```python
from build123d import *

# Parameters (mm, degrees)
BOSS_EXTRUDE1_DEPTH = 50
SKETCH2_W           = 20
SKETCH2_H           = 40
CUT_EXTRUDE1_DEPTH  = 50


with BuildPart() as part:
    # Sketch1 → Boss-Extrude1 (new body)
    with BuildSketch(Plane(origin=(0, 0, 0), x_dir=(1, 0, 0), z_dir=(0, 1, 0))):
        Polygon((40, -2.5), (40, 0), (40, 2.5), (-40, 2.5), (-40, -2.5), align=None)
    extrude(amount=BOSS_EXTRUDE1_DEPTH)

    # Sketch2 → Cut-Extrude1 (cut)
    with BuildSketch(Plane.XY.offset(2.5)):
        with Locations((10, 30)):
            Rectangle(SKETCH2_W, SKETCH2_H)
        with Locations((-10, 30)):
            Rectangle(SKETCH2_W, SKETCH2_H)
    extrude(amount=-CUT_EXTRUDE1_DEPTH, mode=Mode.SUBTRACT)


solid = part.part
```
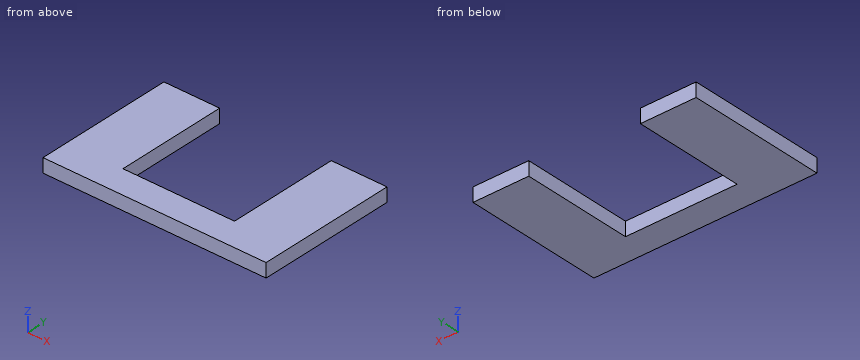
Design review of the part built by this model. Coordinates are the model's own, in mm. Round coordinates to 2 decimals unless told otherwise and drop trailing zeros. Write each loop counter-clockwise with the first axis right and the second up, starting at its lowest first coordinate (ties: lowest second). Pieces come first, ordered by that corner, then holes. Notation, with made-up numbers: (-25.5, -6.75) -> (20.5, -6.75) arc R17 cw to (20.5, -0.75) -> close; hole circle Ø1 at (84.25, 29). An arc over 180 degrees is marked (long way). Answer in a Markdown table with one row per item.
Q1. Take a section at C-C, the plane x = 3. State the section outline as (y, z) points, then the cut area to 3 significant figures.
The answers:
| item | result |
|---|---|
| outline | (0, -2.5) -> (10, -2.5) -> (10, 2.5) -> (0, 2.5) -> close |
| area | 50.0 mm² |
Q2. Take a section at B-B, the plane z = 1.35. State the section outline as (x, y) points.
The answers:
| item | result |
|---|---|
| outline | (-40, 0) -> (40, 0) -> (40, 50) -> (20, 50) -> (20, 10) -> (-20, 10) -> (-20, 50) -> (-40, 50) -> close |
Q3. To check wall thickness, follow L1, parallel to X at y = 21, z = -1.05; L2, parallel to Y at x = 8, z = 0.25. State the ranges of each line that lie inside material, in increasing order. Write a range as [from, to].
The answers:
| item | result |
|---|---|
| L1 | [-40, -20], [20, 40] |
| L2 | [0, 10] |
Q4. Clearance check with flat-ended pins moving along their axes: pin 1 Ø3 at (x, z) = (-5, -1.5) entering from +Y; pin 2 Ø2 at (x, z) = (-2.5, 0) entering from -Y. State where each tip first meets the part, or that it passes through.
The answers:
| item | result |
|---|---|
| pin 1 | y = 10 |
| pin 2 | y = 0 |
Q5. Take a section at A-A, the plane y = 45. State the section outline as (x, z) points.
The answers:
| item | result |
|---|---|
| outline | (-40, -2.5) -> (-20, -2.5) -> (-20, 2.5) -> (-40, 2.5) -> close; (20, -2.5) -> (40, -2.5) -> (40, 2.5) -> (20, 2.5) -> close |
